```python
from build123d import *

# Parameters (mm, degrees)
SKETCH1_R           = 5.05
BOSS_EXTRUDE1_DEPTH = 10
CUT_EXTRUDE1_DEPTH  = 10


with BuildPart() as part:
    # Sketch1 → Boss-Extrude1 (new body)
    with BuildSketch(Plane(origin=(0, 0, 0), x_dir=(1, 0, 0), z_dir=(0, 1, 0))):
        with BuildLine():
            Line((13.338907001, -11.489526472), (11.034706991, 21.319990694))
            ThreePointArc((11.034706991, 21.319990694), (26.944443341, 30.280165305), (9.790047406, 36.535654086))
            ThreePointArc((9.790047406, 36.535654086), (2.201013528, 43.799487348), (-7.715302177, 40.332011077))
            ThreePointArc((-7.715302177, 40.332011077), (-22.969610395, 32.582266479), (-9.193128161, 22.435296597))
            Line((-9.193128161, 22.435296597), (-6.711707001, -12.897673528))
            ThreePointArc((-6.711707001, -12.897673528), (4.017673528, -22.218907001), (13.338907001, -11.489526472))
        make_face()
        with Locations(Location((3.3136, -12.1936, 0), (0, 0, 270))):
            Circle(SKETCH1_R, mode=Mode.SUBTRACT)
        with Locations(Location((-12.9537, 31.7552, 0), (0, 0, 270))):
            Circle(SKETCH1_R, mode=Mode.SUBTRACT)
        with Locations(Location((0.071, 33.9778, 0), (0, 0, 270))):
            Circle(SKETCH1_R, mode=Mode.SUBTRACT)
        with Locations(Location((16.9279, 29.4608, 0), (0, 0, 270))):
            Circle(SKETCH1_R, mode=Mode.SUBTRACT)
    extrude(amount=BOSS_EXTRUDE1_DEPTH)

    # Sketch2 → Cut-Extrude1 (cut)
    with BuildSketch(Plane(origin=(0, 10, 0), x_dir=(1, 0, 0), z_dir=(0, 1, 0))):
        Polygon((-3.820842932, 18.023387052), (6.15458692, 18.723957726), (7.205442932, 3.760812948), (-2.76998692, 3.060242274), align=None)
    extrude(amount=-CUT_EXTRUDE1_DEPTH, mode=Mode.SUBTRACT)


solid = part.part
```
Design review of the part built by this model. Coordinates are the model's own, in mm. A direction names the side the tool comes from. Round coordinates to 2 decimals unless told otherwise and drop trailing zeros. Write each loop counter-clockwise with the first axis right and the second up, starting at its lowest first coordinate (ties: lowest second). Pieces come first, ordered by that corner, then holes. Notation, with made-up numbers: (86, -28) -> (105, -28) arc R27 cw to (105, 7) -> close; hole circle Ø3 at (64.25, -14). An arc over 180 degrees is marked (long way). Answer in a Markdown table with one row per item.
Q1. Clearance check with flat-ended pins moving along their axes: pin 1 Ø6 at (y, z) = (8.5, 2.5) entering from +X; pin 2 Ø8 at (x, z) = (3.31, 12.19) entering from -Y; pin 3 Ø12 at (x, z) = (12.5, -29.5) entering from -Y; pin 4 Ø6 at (y, z) = (6, -20) entering from +X. State where each tip first meets the part, or that it passes through.
The answers:
| item | result |
|---|---|
| pin 1 | x = 12.92 |
| pin 2 | through |
| pin 3 | y = 0 |
| pin 4 | x = 24.63 |
Q2. Take a section at C-C, the plane y = 2. State the section outline as (x, z) points.
The answers:
| item | result |
|---|---|
| outline | (-9.19, -22.44) arc R10.05 ccw (long way) to (-7.72, -40.33) arc R10.05 ccw to (9.79, -36.54) arc R10.05 ccw (long way) to (11.03, -21.32) -> (13.34, 11.49) arc R10.05 ccw to (-6.71, 12.9) -> close; hole circle Ø10.1 at (-12.95, -31.76); hole circle Ø10.1 at (0.07, -33.98); hole (-3.82, -18.02) -> (6.15, -18.72) -> (7.21, -3.76) -> (-2.77, -3.06) -> close; hole circle Ø10.1 at (3.31, 12.19); hole circle Ø10.1 at (16.93, -29.46) |
Q3. For faces 4 (the face through (-3.29, 5.07, -10.44)), 5 (the face through (2, 10, -19)), list the 3-axis set-ups (+Z, -Z, +X, -X, +Y, -Y) from which the entire face can be reached by the end or side of a thin tool; tool diameter is ignored.
The answers:
| item | result |
|---|---|
| face 4 | +Y, -Y |
| face 5 | +Z, -Z, +X, -X, +Y |
Q4. Draft analysis for pull direction Z (two halves, no side actions). For faces 1 (the face through (-7.97, 4.93, -5.02)), 2 (the face through (2, 0, -19)), 3 (the face through (-11.437, 4.93, -26.938)), state which applies: +Z half, -Z half, draft (parallel to the pull), parting line (faces both ways), or undercut.
The answers:
| item | result |
|---|---|
| face 1 | +Z half |
| face 2 | draft |
| face 3 | undercut |
Q5. To check wall thickness, follow L1, parallel to Z at x = -13, y = 8.25; L2, parallel to X at y = 5.75, z = -31; L3, parallel to X at y = 1.5, z = -35.5. State the ranges of each line that lie inside material, in increasing order. Write a range as [from, to].
The answers:
| item | result |
|---|---|
| L1 | [-41.81, -36.8], [-26.71, -21.71] |
| L2 | [-22.98, -17.95], [-7.96, -4.01], [4.15, 12.12], [21.74, 26.86] |
| L3 | [-22.28, -16.34], [-9.57, -4.74], [4.89, 24.96] |
Q6. Take a section at A-A, the plane x = -15.5. State the section outline as (y, z) points, then the cut area to 3 significant figures.
The answers:
| item | result |
|---|---|
| outline | (0, -41.48) -> (10, -41.48) -> (10, -36.12) -> (0, -36.12) -> close; (0, -27.39) -> (10, -27.39) -> (10, -22.03) -> (0, -22.03) -> close |
| area | 107 mm² |
Q7. Take a section at D-D, the plane z = -17. State the section outline as (x, y) points, then the cut area to 3 significant figures.
The answers:
| item | result |
|---|---|
| outline | (-8.81, 0) -> (-3.75, 0) -> (-3.75, 10) -> (-8.81, 10) -> close; (6.28, 0) -> (11.34, 0) -> (11.34, 10) -> (6.28, 10) -> close |
| area | 101 mm² |
Q8. Take a section at B-B, the plane z = -33.5. State the section outline as (x, y) points.
The answers:
| item | result |
|---|---|
| outline | (-22.85, 0) -> (-17.69, 0) -> (-17.69, 10) -> (-22.85, 10) -> close; (-8.21, 0) -> (-4.96, 0) -> (-4.96, 10) -> (-8.21, 10) -> close; (5.1, 0) -> (13.9, 0) -> (13.9, 10) -> (5.1, 10) -> close; (19.96, 0) -> (26.13, 0) -> (26.13, 10) -> (19.96, 10) -> close |
